```python
from build123d import *

# Parameters (mm, degrees)
CROQUIS1_W              = 23.7
CROQUIS1_H              = 44.7
CROQUIS1_W_2            = 20
CROQUIS1_H_2            = 41
SALIENTE_EXTRUIR1_DEPTH = 30.3
CROQUIS1_2_W            = 20
CROQUIS1_2_H            = 41
SALIENTE_EXTRUIR2_DEPTH = 2
SALIENTE_EXTRUIR3_START = 30.3
CROQUIS1_4_W            = 33
CROQUIS1_4_H            = 54
CROQUIS1_4_W_2          = 23.7
CROQUIS1_4_H_2          = 44.7
SALIENTE_EXTRUIR3_DEPTH = 5
CROQUIS2_W              = 23.7
CROQUIS2_H              = 74.7
CROQUIS2_R              = 1.5
SALIENTE_EXTRUIR5_DEPTH = 28.5
REDONDEO2_R             = 5
CORTAR_EXTRUIR1_DEPTH   = 5
CROQUIS4_R              = 2.15
CORTAR_EXTRUIR2_DEPTH   = 10


with BuildPart() as part:
    # Croquis1 → Saliente-Extruir1 (new body)
    with BuildSketch(Plane(origin=(0, 0, 0), x_dir=(1, 0, 0), z_dir=(0, 1, 0))):
        Rectangle(CROQUIS1_W, CROQUIS1_H)
        Rectangle(CROQUIS1_W_2, CROQUIS1_H_2, mode=Mode.SUBTRACT)
    extrude(amount=SALIENTE_EXTRUIR1_DEPTH)

    # Croquis1<2> → Saliente-Extruir2 (add)
    with BuildSketch(Plane(origin=(0, 0, 0), x_dir=(1, 0, 0), z_dir=(0, 1, 0))):
        Rectangle(CROQUIS1_2_W, CROQUIS1_2_H)
    extrude(amount=SALIENTE_EXTRUIR2_DEPTH)

    # Croquis1<4> → Saliente-Extruir3 (add)
    with BuildSketch(Plane(origin=(0, 0, 0), x_dir=(1, 0, 0), z_dir=(0, 1, 0)).offset(SALIENTE_EXTRUIR3_START)):
        Rectangle(CROQUIS1_4_W, CROQUIS1_4_H)
        Rectangle(CROQUIS1_4_W_2, CROQUIS1_4_H_2, mode=Mode.SUBTRACT)
    extrude(amount=-SALIENTE_EXTRUIR3_DEPTH)

    # Croquis2 → Saliente-Extruir5 (add)
    with BuildSketch(Plane.XZ):
        Rectangle(CROQUIS2_W, CROQUIS2_H)
        with Locations((-6.5, 29.85)):
            Circle(CROQUIS2_R, mode=Mode.SUBTRACT)
        with Locations((6.5, 29.85)):
            Circle(CROQUIS2_R, mode=Mode.SUBTRACT)
        with Locations((6.5, -29.85)):
            Circle(CROQUIS2_R, mode=Mode.SUBTRACT)
        with Locations((-6.5, -29.85)):
            Circle(CROQUIS2_R, mode=Mode.SUBTRACT)
    extrude(amount=SALIENTE_EXTRUIR5_DEPTH)

    # Redondeo2
    redondeo2_edges = [part.edges().sort_by_distance(p)[0] for p in [
        (0, 0, 22.35),
        (0, 0, -22.35),
    ]]
    fillet(redondeo2_edges, radius=REDONDEO2_R)

    # Croquis3 → Cortar-Extruir1 (cut, symmetric)
    with BuildSketch(Plane.XY.offset(22.35)):
        with BuildLine():
            Line((-2.325, 9.325), (2.325, 9.325))
            ThreePointArc((2.325, 9.325), (2.926040764, 9.076040764), (3.175, 8.475))
            Line((3.175, 8.475), (3.175, 6.625))
            ThreePointArc((3.175, 6.625), (2.926040764, 6.023959236), (2.325, 5.775))
            Line((2.325, 5.775), (-2.325, 5.775))
            ThreePointArc((-2.325, 5.775), (-2.926040764, 6.023959236), (-3.175, 6.625))
            Line((-3.175, 6.625), (-3.175, 8.475))
            ThreePointArc((-3.175, 8.475), (-2.926040764, 9.076040764), (-2.325, 9.325))
        make_face()
    extrude(amount=CORTAR_EXTRUIR1_DEPTH, both=True, mode=Mode.SUBTRACT)

    # Croquis4 → Cortar-Extruir2 (cut)
    with BuildSketch(Plane(origin=(0, 30.3, 0), x_dir=(1, 0, 0), z_dir=(0, 1, 0))):
        with Locations((-4.85, 24.55)):
            Circle(CROQUIS4_R)
        with Locations((4.85, 24.55)):
            Circle(CROQUIS4_R)
        with Locations((-4.85, -24.55)):
            Circle(CROQUIS4_R)
        with Locations((4.85, -24.55)):
            Circle(CROQUIS4_R)
    extrude(amount=-CORTAR_EXTRUIR2_DEPTH, mode=Mode.SUBTRACT)


solid = part.part
```
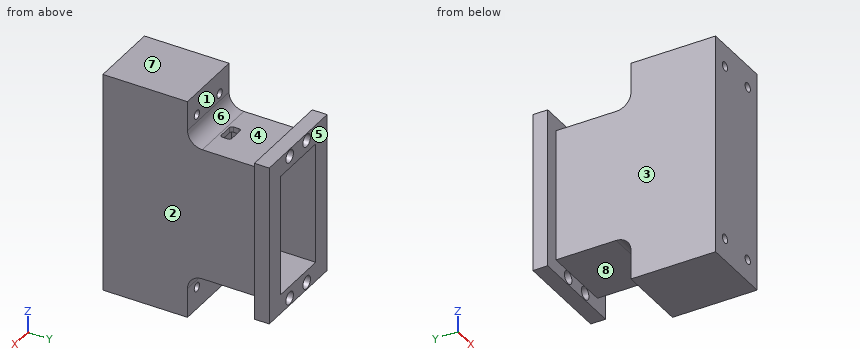
Build history of the part. All positions in model axes, mm. Face numbers are marked on the shaded views. A direction names the side the tool comes from. Give positions to 0.01 mm unless a question says otherwise; leave off trailing zeros. Loops run counter-clockwise (first coordinate to the right, second up) from the corner with the lowest first, then second, coordinate; pieces in that order, holes last. Notation, with made-up numbers: (15, 29.5) -> (73, 29.5) arc R38 cw to (73, 68.5) -> close; hole circle Ø2 at (63, 2.25). An arc over 180 degrees is marked (long way). One line per question, with ' | ' between items. Start each with the question number.
1) Cut at A-A (z = -29.85). Give the cut face in (x, y).
2) Probe L1, parallel to X at y = 29.25, z = -24.55; L2, parallel to Z at x = 6.5, y = -14.5; L3, parallel to Z at x = -4.85, y = 28.4. List the from-to ranges inside material, lowest first.
3) Two-plate mould, pull along Y, no slides. Class the marked faces 5, 6, 7 and 8: released by +Y, released by -Y, zero draft, split by the parting line, or undercut.
4) Cut at D-D (y = -17.5). Give the cut face in (x, z), plus the area to 3 significant figures.
5) 3-axis set-ups, long thin cutter, end or side, ignore diameter. For the marked faces 1, 2, 3 and 4: which of +Z, -Z, +X, -X, +Y, -Y reach the whole face in a straight line?
6) Cut at C-C (x = -1.5). Give the cut face in (y, z) (3 decimals), plus the area to 3 significant figures.
7) Pin check, flat tips, straight feed: pin 1 (4 mm diameter, centred on y = 11.5, z = 5.5, fed in from -X); pin 2 (8 mm diameter, centred on y = -14.5, z = 19.5, fed in from +X); pin 3 (2.5 mm diameter, centred on x = 4.85, z = 24.55, fed in from +Y). Stop position of each tip, or through.
8) Cut at B-B (y = 11). Give the cut face in (x, z).
Return value:
1) outline: (-11.85, -28.5) -> (-8, -28.5) -> (-8, 0) -> (-11.85, 0) -> close; (-5, -28.5) -> (5, -28.5) -> (5, 0) -> (-5, 0) -> close; (8, -28.5) -> (11.85, -28.5) -> (11.85, 0) -> (8, 0) -> close
2) L1: -16.5 to -7, -2.7 to 2.7, 7 to 16.5 | L2: -37.35 to -31.35, -28.35 to 28.35, 31.35 to 37.35 | L3: -27 to -26.7, -22.4 to -20.5, 20.5 to 22.4, 26.7 to 27
3) face 5: released by +Y | face 6: undercut | face 7: zero draft | face 8: undercut
4) outline: (-11.85, -37.35) -> (11.85, -37.35) -> (11.85, 37.35) -> (-11.85, 37.35) -> close; hole circle Ø3 at (-6.5, -29.85); hole circle Ø3 at (-6.5, 29.85); hole circle Ø3 at (6.5, -29.85); hole circle Ø3 at (6.5, 29.85) | area: 1,740 mm^2
5) face 1: +Z, +X, -X, +Y | face 2: +Z, -Z, +X, -Y | face 3: +Z, -Z, -X, -Y | face 4: +Z, +X, -X
6) outline: (-28.5, -37.35) -> (0, -37.35) -> (0, -27.35) arc R5 cw to (5, -22.35) -> (25.3, -22.35) -> (25.3, -27) -> (30.3, -27) -> (30.3, -20.5) -> (2, -20.5) -> (2, 20.5) -> (5.775, 20.5) -> (5.775, 22.35) -> (5, 22.35) arc R5 cw to (0, 27.35) -> (0, 37.35) -> (-28.5, 37.35) -> close; (9.325, 20.5) -> (30.3, 20.5) -> (30.3, 27) -> (25.3, 27) -> (25.3, 22.35) -> (9.325, 22.35) -> close | area: 2,370 mm^2
7) pin 1: x = -11.85 | pin 2: x = 11.85 | pin 3: y = 2.07
8) outline: (-11.85, -22.35) -> (11.85, -22.35) -> (11.85, 22.35) -> (-11.85, 22.35) -> close; hole (-10, -20.5) -> (10, -20.5) -> (10, 20.5) -> (-10, 20.5) -> close
